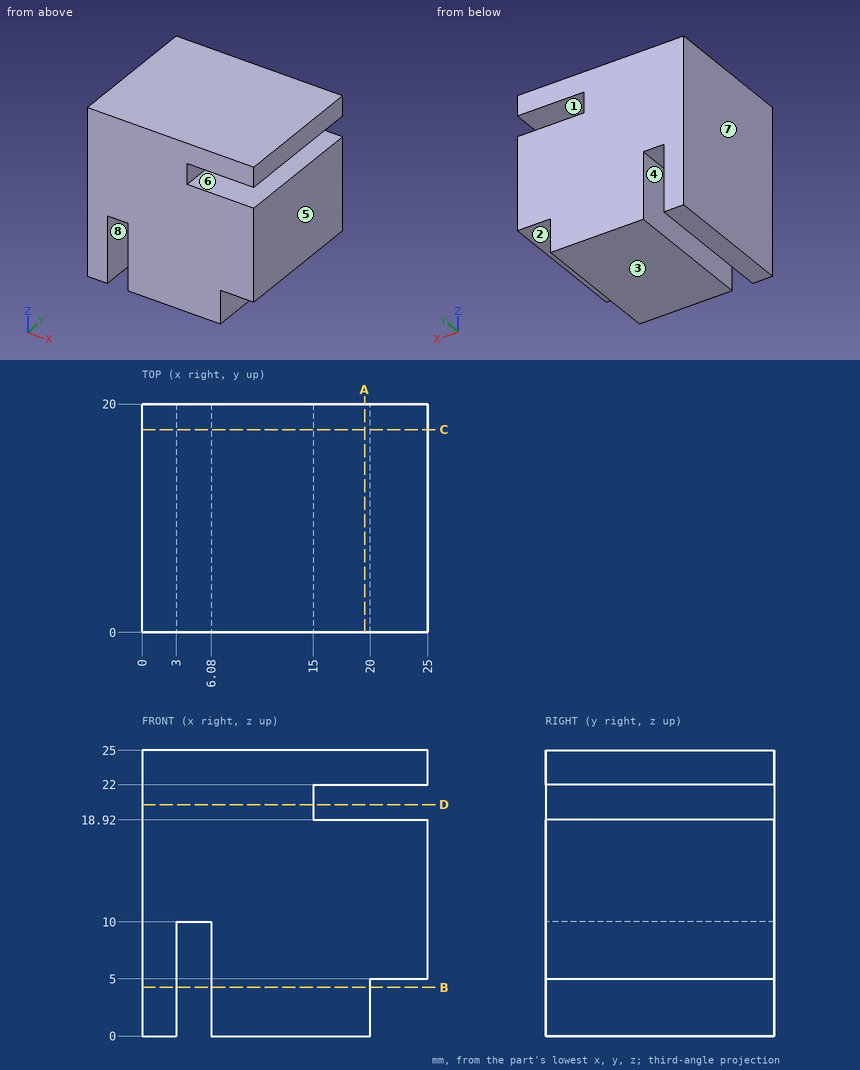
Answer from the drawing. Dimensions are ordinates in mm from the lowest x, y and z of the part. A direction names the side the tool comes from. Give positions to 0.01 mm unless a question says otherwise; leave off trailing zeros. Order: outer loops, then holes, each group sorted by start corner. A loop starts at its lowest first (then second) coordinate and runs counter-clockwise, first axis right, second up.
Item 1: The part is cut by section D-D, the plane z = 20.25. Give the vertices of the cut face in (x, y).
From the geometry:
outline: (0, 0) - (15, 0) - (15, 20) - (0, 20) - close
Item 2: For a pull along X with two mould halves and no side action, classify the marked faces 5, 6, 7 and 8 as pulls with the +X half, pulls with the -X half, needs draft (parallel to the pull), parting line crosses it, or undercut.
From the geometry:
face 5: pulls with the +X half
face 6: needs draft
face 7: pulls with the -X half
face 8: undercut
Item 3: Find the intervals of material crossed by probe 1 along X at (y, z) = (16, 3.25); probe 2 along Z at (x, y) = (22.25, 7); probe 3 along Z at (x, y) = (4.5, 11.75), in increasing order.
From the geometry:
probe 1: x = 0 to 3, 6.08 to 20
probe 2: z = 5 to 18.92, 22 to 25
probe 3: z = 10 to 25
Item 4: The part is cut by section B-B, the plane z = 4.25. Give the vertices of the cut face in (x, y), and give its area (3 significant figures).
From the geometry:
outline: (0, 0) - (3, 0) - (3, 20) - (0, 20) - close; (6.08, 0) - (20, 0) - (20, 20) - (6.08, 20) - close
area: 338 mm2
Item 5: The part is cut by section A-A, the plane x = 19.5. Give the vertices of the cut face in (y, z), and give its area (3 significant figures).
From the geometry:
outline: (0, 0) - (20, 0) - (20, 18.92) - (0, 18.92) - close; (0, 22) - (20, 22) - (20, 25) - (0, 25) - close
area: 438 mm2
Item 6: The part is cut by section C-C, the plane y = 17.75. Give the vertices of the cut face in (x, z), and give its area (3 significant figures).
From the geometry:
outline: (0, 0) - (3, 0) - (3, 10) - (6.08, 10) - (6.08, 0) - (20, 0) - (20, 5) - (25, 5) - (25, 18.92) - (15, 18.92) - (15, 22) - (25, 22) - (25, 25) - (0, 25) - close
area: 538 mm2
Item 7: Given pin 1 Ø8 at (x, y) = (3.5, 16) entering from -Z; pin 2 Ø0.9 at (y, z) = (12, 21) entering from +X; pin 3 Ø1.5 at (x, y) = (5, 6) entering from -Z; pin 4 Ø5.5 at (y, z) = (8.5, 1.5) entering from +X, each flat-ended and moving along its own axis, determine where each tip first touches the part or whether it passes through.
From the geometry:
pin 1: stops at z = 0
pin 2: stops at x = 15
pin 3: stops at z = 10
pin 4: stops at x = 20
Item 8: Which of the six approach directions +Z, -Z, +X, -X, +Y, -Y give full straight-line access (tool end or side, diameter ignored) to the marked faces 1, 2, 3 and 4?
From the geometry:
face 1: +X, +Y, -Y
face 2: -Z, +X, +Y, -Y
face 3: -Z, +X, -X, +Y, -Y
face 4: -Z, +Y, -Y
